Autodesk Inventor part; units mm, degrees
ref_plane "YZ Plane" through (0, 0, 0) normal (1, 0, 0) x (0, 1, 0)
ref_plane "XZ Plane" through (0, 0, 0) normal (0, 1, 0) x (-1, 0, 0)
ref_plane "XY Plane" through (0, 0, 0) normal (0, 0, 1) x (1, 0, 0)
sketch "Sketch1" plane through (0, 0, 0) normal (0, 1, 0) x (-1, 0, 0)
  line L0 (14.605, 14.605) -> (-14.605, 14.605)
  line L1 (-14.605, 14.605) -> (-14.605, -14.605)
  line L2 (-14.605, -14.605) -> (14.605, -14.605)
  line L3 (14.605, -14.605) -> (14.605, 14.605)
  point P0 (0, 0)
  point P1 (14.605, 0)
  point P2 (0, -14.605)
  dimension "d0" = 29.21
  dimension "d1" = 29.21
extrude "Extrusion1" add sketch "Sketch1" along normal blind 2.54
sketch "Sketch2" plane through (0, 2.54, 0) normal (0, 1, 0) x (1, 0, 0)
  line L0 (-12.7, -12.7) -> (12.7, -12.7)
  line L1 (12.7, -12.7) -> (12.7, 12.7)
  line L2 (12.7, 12.7) -> (-12.7, 12.7)
  line L3 (-12.7, 12.7) -> (-12.7, -12.7)
  point P0 (0, 0)
  point P1 (0, 12.7)
  point P2 (-12.7, 0)
  dimension "d4" = 25.4
  dimension "d5" = 25.4
extrude "Extrusion2" add sketch "Sketch2" along normal blind 5.08
sketch "Sketch3" plane through (0, 7.62, 0) normal (0, 1, 0) x (1, 0, 0)
  line L0 (0, 0) -> (0, 11.557)
  line L1 (0, 11.557) -> (0, -11.557)
  line L2 (0, -11.557) -> (0, -11.0469)
  line L3 (0, 0) -> (-10.795, 0)
  line L4 (-10.795, 0) -> (10.795, 0)
  line L5 (0, -11.557) -> (-10.795, -11.557)
  line L6 (-10.795, -11.557) -> (-10.795, 11.557)
  line L7 (-10.795, 11.557) -> (0, 11.557)
  line L8 (10.795, 0) -> (10.795, 6)
  line L9 (10.795, 6) -> (10.795, -6)
  line L10 (10.795, -6) -> (0, -11.557)
  line L11 (10.795, 6) -> (0, 11.557)
  dimension "d8" = 11.557
  dimension "d9" = 23.114
  dimension "d10" = 10.795
  dimension "d11" = 21.59
  dimension "d12" = 6
  dimension "d13" = 12
extrude "Extrusion3" cut sketch "Sketch3" against normal blind 25.4
properties part number "Adapter_3DPrint"
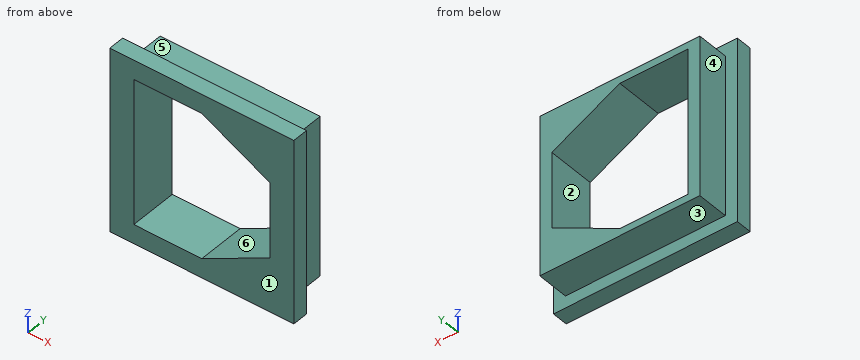
For this review, take the finished solid that the model builds, in its own axes (mm). Face numbers are marked on the shaded views. A direction names the side the tool comes from. Round coordinates to 2 decimals unless told otherwise and drop trailing zeros. Order: outer loops, then holes, each group sorted by start corner. A loop starts at its lowest first (then second) coordinate and runs counter-clockwise, first axis right, second up.
Q1. We need section A-A, the plane z = -0.5. Give the boundary of the cut face in (x, y) (3 decimals).
Findings below:
outline: (-14.605, 0) - (-10.795, 0) - (-10.795, 7.62) - (-12.7, 7.62) - (-12.7, 2.54) - (-14.605, 2.54) - close; (10.795, 0) - (14.605, 0) - (14.605, 2.54) - (12.7, 2.54) - (12.7, 7.62) - (10.795, 7.62) - close
Q2. Mouldability with a two-part tool opening along Z and no side actions: class the marked faces 4, 5 and 6 as pulls with the +Z half, pulls with the -Z half, needs draft (parallel to the pull), parting line crosses it, or undercut.
Findings below:
face 4: needs draft
face 5: pulls with the +Z half
face 6: undercut
Q3. Wall thickness on line 1 (X direction, y = 3.25, z = 2.5) (3 decimals); line 2 (Z direction, x = -8, y = 5.5); line 3 (X direction, y = 0.5, z = -2.5) (3 decimals): over which ranges is each line inside the solid? List them lowest first.
Findings below:
line 1: x = -12.7 to -10.795, 10.795 to 12.7
line 2: z = -12.7 to -11.56, 11.56 to 12.7
line 3: x = -14.605 to -10.795, 10.795 to 14.605
Q4. We need section B-B, the plane y = 5.25. Give the boundary of the cut face in (x, z) (3 decimals).
Findings below:
outline: (-12.7, -12.7) - (12.7, -12.7) - (12.7, 12.7) - (-12.7, 12.7) - close; hole (-10.795, -11.557) - (0, -11.557) - (10.795, -6) - (10.795, 6) - (0, 11.557) - (-10.795, 11.557) - close
Q5. Insertion check: P1, Ø8, axis at x = -2.5, z = -10.5, coming from the -Y side; P2, Ø2.5, axis at x = -0.5, y = 4.5, coming from the -Z side; P3, Ø1, axis at x = 10.5, y = 5, coming from the +Z side; P4, Ø1.5, axis at y = 4, z = -1, coming from the +X side. Each pin has a flat end and moves straight along its axis. Give the tip position at first contact, or say it passes through.
Findings below:
P1: stops at y = 0
P2: stops at z = -12.7
P3: stops at z = 12.7
P4: stops at x = 12.7
Q6. Machinability: for the marked faces 1, 2 and 3, which of the approach directions +Z, -Z, +X, -X, +Y, -Y give a long, thin tool a straight path to every point of the face, cutting with its end or side? Answer none if there is none.
Findings below:
face 1: +Z, -Z, +X, -X, -Y
face 2: +Y, -Y
face 3: -Z, +X, -X, +Y
Q7. We need section C-C, the plane x = -6.75. Give the boundary of the cut face in (y, z) (3 decimals).
Findings below:
outline: (0, -14.605) - (2.54, -14.605) - (2.54, -12.7) - (7.62, -12.7) - (7.62, -11.557) - (0, -11.557) - close; (0, 11.557) - (7.62, 11.557) - (7.62, 12.7) - (2.54, 12.7) - (2.54, 14.605) - (0, 14.605) - close
Q8. We need section D-D, the plane x = 11.75. Give the boundary of the cut face in (y, z) (3 decimals).
Findings below:
outline: (0, -14.605) - (2.54, -14.605) - (2.54, -12.7) - (7.62, -12.7) - (7.62, 12.7) - (2.54, 12.7) - (2.54, 14.605) - (0, 14.605) - close
